```python
from build123d import *

# Parameters (mm, degrees)
PAD_DEPTH       = 50
SKETCH001_W     = 30
SKETCH001_H     = 20
POCKET_DEPTH    = 50.001
POCKET001_DEPTH = 60.001
SKETCH003_R     = 15
POCKET002_DEPTH = 50.001


with BuildPart() as part:
    # Sketch → Pad (new body)
    with BuildSketch(Plane.XY):
        with BuildLine():
            Line((0, 30), (90, 30))
            Line((90, 30), (90, -30))
            Line((90, -30), (0, -30))
            ThreePointArc((0, 30), (-29.999955, 0), (0, -30))
        make_face()
    extrude(amount=PAD_DEPTH)

    # Sketch001 (on Face6 of Pad) → Pocket (cut, through all)
    with BuildSketch(Plane.XY.offset(50)):
        with Locations((60, 0)):
            Rectangle(SKETCH001_W, SKETCH001_H)
    extrude(amount=-POCKET_DEPTH, mode=Mode.SUBTRACT)

    # Sketch002 (on Face6 of Pocket) → Pocket001 (cut, through all)
    with BuildSketch(Plane.XZ.offset(30)):
        Polygon((30, 50), (90, 50), (90, 10), align=None)
    extrude(amount=-POCKET001_DEPTH, mode=Mode.SUBTRACT)

    # Sketch003 (on Face5 of Pocket001) → Pocket002 (cut, through all)
    with BuildSketch(Plane.XY.offset(50)):
        Circle(SKETCH003_R)
    extrude(amount=-POCKET002_DEPTH, mode=Mode.SUBTRACT)


solid = part.part
```
Verification items for the finished model (mm, model axes). A direction names the side the tool comes from. Round coordinates to 2 decimals unless told otherwise and drop trailing zeros. Order: outer loops, then holes, each group sorted by start corner. A loop starts at its lowest first (then second) coordinate and runs counter-clockwise, first axis right, second up. Notation, with made-up numbers: (-3, -13.5) -> (24, -13.5) arc R18 cw to (24, -8.5) -> close; hole circle Ø7 at (62.25, -1.75). An arc over 180 degrees is marked (long way). Put each result on its own line as item: value. Start each with the question number.
(1) Material ranges on line 1 along X through (y, z) = (-13, 23.5); line 2 along X through (y, z) = (-5, 11.5); line 3 along X through (y, z) = (-1.5, 22.5), recorded low to high.
(2) Depth check by flat-ended pin: pin 1 Ø5 at (y, z) = (-1, 18) entering from -X; pin 2 Ø8 at (y, z) = (-21, 34.5) entering from -X; pin 3 Ø1 at (y, z) = (12, 42.5) entering from +X. Enter the tip coordinate at first touch or a pass-through.
(3) Section check D-D (x = -3). Enter the section's corners in (y, z), then the cut area to 3 significant figures.
(4) Section check C-C (z = 30). Enter the section's corners in (x, y), then the cut area to 3 significant figures.
(5) Section check A-A (y = 0). Enter the section's corners in (x, z), then the cut area to 3 significant figures.
(6) Section check B-B (z = 18). Enter the section's corners in (x, y).
(7) Draft check along X on faces 3 (the face through (60, -14, 30)), 4 (the face through (60, -10, 16)), 5 (the face through (34, 30, 19)). Enter one of: +X half, -X half, draft (parallel to the pull), parting line (faces both ways), or undercut.
(8) Tool access check on faces 1 (the face through (45, 0, 20)), 2 (the face through (-29.993, 0.66, 24.65)). Record the directions out of +Z, -Z, +X, -X, +Y, -Y that give a thin tool (end or side, any length) a straight path to the whole face; none if there is none.
Completed:
1. line 1: x = -27.04 to -7.48, 7.48 to 69.75
1. line 2: x = -29.58 to -14.14, 14.14 to 45, 75 to 87.75
1. line 3: x = -29.96 to -14.92, 14.92 to 45
2. pin 1: stops at x = -30
2. pin 2: stops at x = -24.72
2. pin 3: stops at x = 42
3. outline: (-29.85, 0) -> (-14.7, 0) -> (-14.7, 50) -> (-29.85, 50) -> close; (14.7, 0) -> (29.85, 0) -> (29.85, 50) -> (14.7, 50) -> close
3. area: 1,520 mm2
4. outline: (0, -30) -> (60, -30) -> (60, -10) -> (45, -10) -> (45, 10) -> (60, 10) -> (60, 30) -> (0, 30) arc R30 ccw to start; hole circle Ø30 at (0, 0)
4. area: 4,010 mm2
5. outline: (-30, 0) -> (-15, 0) -> (-15, 50) -> (-30, 50) -> close; (15, 0) -> (45, 0) -> (45, 40) -> (30, 50) -> (15, 50) -> close; (75, 0) -> (90, 0) -> (90, 10) -> (75, 20) -> close
5. area: 2,400 mm2
6. outline: (0, -30) -> (78, -30) -> (78, 30) -> (0, 30) arc R30 ccw to start; hole circle Ø30 at (0, 0); hole (45, -10) -> (75, -10) -> (75, 10) -> (45, 10) -> close
7. face 3: +X half
7. face 4: undercut
7. face 5: draft
8. face 1: +Z, -Z
8. face 2: +Z, -Z, -X
